Geometry: final body of the model. Coordinates: model frame, mm. A direction names the side the tool comes from. Give positions to 0.01 mm unless a question says otherwise; leave off trailing zeros. Loops run counter-clockwise (first coordinate to the right, second up) from the corner with the lowest first, then second, coordinate; pieces in that order, holes last. Notation, with made-up numbers: (71, 19) - (94, 19) arc R25 cw to (94, 55) - close; hole circle Ø1 at (-25.75, 20.25). An arc over 180 degrees is marked (long way). Use one line per item in the form item = value.
```python
from build123d import *

# Parameters (mm, degrees)
SKETCH1_R           = 60
SKETCH1_R_2         = 1.1
BOSS_EXTRUDE1_DEPTH = 3
SKETCH2_W           = 5.018752931
SKETCH2_H           = 3
CUT_EXTRUDE1_DEPTH  = 1.5
CIRPATTERN1_COUNT   = 3
CUT_EXTRUDE2_REACH  = 91.692
FILLET1_R           = 3


with BuildPart() as part:
    # Sketch1 → Boss-Extrude1 (new body)
    with BuildSketch(Plane(origin=(0, 63.433902084, 0), x_dir=(1, 0, 0), z_dir=(0, 1, 0))):
        with Locations(Location((0, 6.619681527, 0), (0, 0, 270))):
            Circle(SKETCH1_R)
        with Locations(Location((-8.75, 6.619681527, 0), (0, 0, 270))):
            Circle(SKETCH1_R_2, mode=Mode.SUBTRACT)
        with Locations(Location((19.05, 6.619681527, 0), (0, 0, 270))):
            Circle(SKETCH1_R_2, mode=Mode.SUBTRACT)
        with BuildLine():
            Line((1.562049935, 12.719681527), (0, 12.719681527))
            Line((0, 12.719681527), (-1.562049935, 12.719681527))
            Line((-1.562049935, 12.719681527), (-5.25, 12.719681527))
            ThreePointArc((-5.25, 12.719681527), (-5.851040764, 12.470722291), (-6.1, 11.869681527))
            Line((-6.1, 11.869681527), (-6.1, 8.181731462))
            Line((-6.1, 8.181731462), (-6.1, 6.619681527))
            Line((-6.1, 6.619681527), (-6.1, 5.057631592))
            Line((-6.1, 5.057631592), (-6.1, 1.369681527))
            ThreePointArc((-6.1, 1.369681527), (-5.851040764, 0.768640763), (-5.25, 0.519681527))
            Line((-5.25, 0.519681527), (-1.562049935, 0.519681527))
            Line((-1.562049935, 0.519681527), (0, 0.519681527))
            Line((0, 0.519681527), (1.562049935, 0.519681527))
            Line((1.562049935, 0.519681527), (15.55, 0.519681527))
            ThreePointArc((15.55, 0.519681527), (16.151040764, 0.768640763), (16.4, 1.369681527))
            Line((16.4, 1.369681527), (16.4, 11.869681527))
            ThreePointArc((16.4, 11.869681527), (16.151040764, 12.470722291), (15.55, 12.719681527))
            Line((15.55, 12.719681527), (1.562049935, 12.719681527))
        make_face(mode=Mode.SUBTRACT)
    extrude(amount=BOSS_EXTRUDE1_DEPTH)

    # Sketch2 → Cut-Extrude1 (cut, symmetric)
    with BuildSketch(Plane(origin=(0, 0, 0), x_dir=(0, 0, -1), z_dir=(1, 0, 0))):
        with Locations((64.110305062, 64.933902084)):
            Rectangle(SKETCH2_W, SKETCH2_H)
    cut_extrude1 = extrude(amount=CUT_EXTRUDE1_DEPTH, both=True, mode=Mode.SUBTRACT)

    # CirPattern1: Cut-Extrude1 ×3 about axis
    cirpattern1_axis = Axis((0, 0, -6.619681527), (0, 1, 0))
    for i in range(1, CIRPATTERN1_COUNT):
        add(cut_extrude1.rotate(cirpattern1_axis, i * 360 / CIRPATTERN1_COUNT), mode=Mode.SUBTRACT)

    # Sketch3 → Cut-Extrude2 (cut, up to next)
    with BuildSketch(Plane(origin=(0, 66.433902084, 0), x_dir=(1, 0, 0), z_dir=(0, 1, 0)), mode=Mode.PRIVATE) as cut_extrude2_sk1:
        with BuildLine():
            Line((35.312079594, -28.778864132), (44.227211632, -33.926018014))
            ThreePointArc((44.227211632, -33.926018014), (0, -53.380318473), (-44.227211632, -33.926018014))
            Line((-44.227211632, -33.926018014), (-35.312079594, -28.778864132))
            ThreePointArc((-35.312079594, -28.778864132), (0, -43.380318473), (35.312079594, -28.778864132))
        make_face()
    cut_extrude2_tool1 = extrude(cut_extrude2_sk1.sketch, amount=-CUT_EXTRUDE2_REACH, mode=Mode.PRIVATE) & part.part
    # Sketch3 → Cut-Extrude2 (cut, up to next)
    with BuildSketch(Plane(origin=(0, 66.433902084, 0), x_dir=(1, 0, 0), z_dir=(0, 1, 0)), mode=Mode.PRIVATE) as cut_extrude2_sk2:
        with BuildLine():
            Line((48.312079594, -6.262203633), (57.227211632, -11.409357515))
            ThreePointArc((57.227211632, -11.409357515), (51.961524227, 36.619681527), (13, 65.194420109))
            Line((13, 65.194420109), (13, 54.900112345))
            ThreePointArc((13, 54.900112345), (43.301270189, 31.619681527), (48.312079594, -6.262203633))
        make_face()
    cut_extrude2_tool2 = extrude(cut_extrude2_sk2.sketch, amount=-CUT_EXTRUDE2_REACH, mode=Mode.PRIVATE) & part.part
    # Sketch3 → Cut-Extrude2 (cut, up to next)
    with BuildSketch(Plane(origin=(0, 66.433902084, 0), x_dir=(1, 0, 0), z_dir=(0, 1, 0)), mode=Mode.PRIVATE) as cut_extrude2_sk3:
        with BuildLine():
            Line((-48.312079594, -6.262203633), (-57.227211632, -11.409357515))
            ThreePointArc((-57.227211632, -11.409357515), (-51.961524227, 36.619681527), (-13, 65.194420109))
            Line((-13, 65.194420109), (-13, 54.900112345))
            ThreePointArc((-13, 54.900112345), (-43.301270189, 31.619681527), (-48.312079594, -6.262203633))
        make_face()
    cut_extrude2_tool3 = extrude(cut_extrude2_sk3.sketch, amount=-CUT_EXTRUDE2_REACH, mode=Mode.PRIVATE) & part.part
    add(cut_extrude2_tool1.solids().sort_by_distance((0, 66.433902, 52.4622))[0], mode=Mode.SUBTRACT)
    add(cut_extrude2_tool2.solids().sort_by_distance((53.21901, 66.433902, 8.057458))[0], mode=Mode.SUBTRACT)
    add(cut_extrude2_tool3.solids().sort_by_distance((-13.898729, 66.433902, -60.047266))[0], mode=Mode.SUBTRACT)

    # Fillet1
    fillet1_edges = [part.edges().sort_by_distance(p)[0] for p in [
        (-13, 64.933902084, -54.900112345),
        (-48.312079594, 64.933902084, 6.262203633),
        (-57.227211632, 64.933902084, 11.409357515),
        (-13, 64.933902084, -65.194420109),
        (-35.312079594, 64.933902084, 28.778864132),
        (35.312079594, 64.933902084, 28.778864132),
        (44.227211632, 64.933902084, 33.926018014),
        (-44.227211632, 64.933902084, 33.926018014),
        (48.312079594, 64.933902084, 6.262203633),
        (13, 64.933902084, -54.900112345),
        (13, 64.933902084, -65.194420109),
        (57.227211632, 64.933902084, 11.409357515),
    ]]
    fillet(fillet1_edges, radius=FILLET1_R)


solid = part.part
```
(1) Access query for faces 5 (the face through (49, 64.955, 23.402)), 6 (the face through (5, 65, -12.72)), 7 (the face through (-1.5, 65, -64)), 8 (the face through (-48.72, 64.91, 28.4)). Directions: +Z, -Z, +X, -X, +Y, -Y. A direction counts if a zero-diameter tool reaches every point of the face in a straight line with its end or side. Return the directions, or none.
Solution:
face_5 = +X, +Y, -Y
face_6 = +Y, -Y
face_7 = -Z, +Y, -Y
face_8 = +Z, -X, +Y, -Y
(2) Cut plane D-D (z = 35). Return the cut outline in (x, y).
Solution:
outline = (-27.71, 63.43) - (27.71, 63.43) - (27.71, 66.43) - (-27.71, 66.43) - close
(3) Cut plane A-A (z = -9). Return the cut outline in (x, y).
Solution:
outline = (-49.94, 63.43) - (-6.1, 63.43) - (-6.1, 66.43) - (-49.94, 66.43) - close; (16.4, 63.43) - (49.94, 63.43) - (49.94, 66.43) - (16.4, 66.43) - close
(4) Material intervals for L1, parallel to X at y = 63.7, z = -6.5; L2, parallel to X at y = 65, z = 30; L3, parallel to Z at x = -0.5, y = 65.45, sorted ascending. Write a range as from..to.
Solution:
L1 = -50..-9.84, -7.66..-6.1, 16.4..17.96, 20.14..50
L2 = -47.53..-37.43, -34.1..34.1, 37.43..47.53
L3 = -61.6..-12.72, -0.52..43.38
(5) Cut plane C-C (x = 29.5). Return the cut outline in (y, z), plus the area to 3 significant figures.
Solution:
outline = (63.43, -46.99) - (66.43, -46.99) - (66.43, 33.75) - (63.43, 33.75) - close
area = 242 mm2
(6) Pin query (flat end, axial travel): P1, Ø3, axis at x = -8.75, z = -6.62, coming from the -Y side; P2, Ø0.9, axis at y = 64.5, z = -63.5, coming from the +X side; P3, Ø1.5, axis at y = 64.5, z = -59.5, coming from the -X side; P4, Ø1.5, axis at y = 65.5, z = -5, coming from the +X side. Return the tip coordinate at first contact, or that it passes through.
Solution:
P1 = 63.43
P2 = 12.98
P3 = -13
P4 = 49.99
(7) Cut plane B-B (y = 65.6). Give the number of separate pieces and of enclosed holes in the cut face, plus the area to 3 significant figures.
Solution:
separate_pieces = 1
enclosed_holes = 3
area = 8,310 mm2
(8) Pull-direction query (X, two-part tool) for faces 1 (the face through (-13, 65, -60)), 2 (the face through (50.5, 64.955, 20.804)), 3 (the face through (16.4, 65, -7)), 4 (the face through (13.56, 64.91, -55.4)); classes: released by +X, released by -X, zero draft, split by the parting line, or undercut.
Solution:
face_1 = released by -X
face_2 = undercut
face_3 = undercut
face_4 = released by +X
